Read the model definition and answer for the solid it produces. Units are mm, in the model's axes. Give positions to 0.01 mm unless a question says otherwise; leave off trailing zeros. Order: outer loops, then holes, each group sorted by start corner. A loop starts at its lowest first (then second) coordinate and runs counter-clockwise, first axis right, second up. Notation, with made-up numbers: (35, 56.25) - (40, 56.25) arc R29 cw to (40, 92.25) - close; hole circle Ø1 at (-8, 9.5). An arc over 180 degrees is marked (long way). Write each question's results on one line, items separated by ' | '.
from build123d import *

# Parameters (mm, degrees)
F0_R     = 35.664624
F1_DEPTH = 76.2
F3_D     = 25.4
F4_R     = 5.08


with BuildPart() as f1:
    # F0 (on Front) → F1 (new body)
    with BuildSketch(Plane.XZ):
        with Locations((-92.187047, 32.669652)):
            Circle(F0_R)
    extrude(amount=-F1_DEPTH)

    # F3 (through all)
    with Locations(Plane.XZ):
        with Locations((-92.187047, 32.669652)):
            Hole(F3_D / 2)

    # F4
    f4_edges = [f1.edges().sort_by_distance(p)[0] for p in [
        (-127.851671, 0, 32.669652),
    ]]
    fillet(f4_edges, radius=F4_R)


solid = f1.part
(1) Each of these flat-tipped pins is pushed along its axis until it touches: pin 1 (6 mm diameter, centred on y = 67.5, z = 14, fed in from -X); pin 2 (2 mm diameter, centred on x = -77.5, y = 28, fed in from -Z); pin 3 (6 mm diameter, centred on y = 30, z = 17.5, fed in from +X). Where does it stop, or does it pass through?
Conclusion:
pin 1: x = -124.22 | pin 2: z = -0.26 | pin 3: x = -58.66
(2) Section A-A (y = 59) is taken. Give the vertices of the cut face in (x, z).
Conclusion:
outline: circle Ø71.33 at (-92.19, 32.67); hole circle Ø25.4 at (-92.19, 32.67)
(3) The mould has two halves that part along X. Classify faces 1 (the face through (-103.92, 38.63, 27.81)), 2 (the face through (-77, 76.2, 33)), 3 (the face through (-120.49, 40.14, 10.97)): pulls with the +X half, pulls with the -X half, needs draft (parallel to the pull), parting line crosses it, or undercut.
Conclusion:
face 1: undercut | face 2: needs draft | face 3: parting line crosses it
(4) Consider probe 1 along Z at (x, y) = (-81, 24); probe 2 along X at (y, z) = (28, 22); probe 3 along Z at (x, y) = (-88.5, 30). Determine where each line is inside the solid, lowest interval first. Write a range as [from, to].
Conclusion:
probe 1: [-1.2, 26.66], [38.68, 66.53] | probe 2: [-126.22, -99.08], [-85.3, -58.16] | probe 3: [-2.8, 20.52], [44.82, 68.14]
